Could you check a few things on this model? Use its own coordinates, in mm. A direction names the side the tool comes from. Round coordinates to 2 decimals unless told otherwise and drop trailing zeros. Write each loop counter-clockwise with the first axis right and the second up, starting at its lowest first coordinate (ties: lowest second). Pieces come first, ordered by that corner, then holes. Notation, with made-up numbers: (84.25, -31) -> (91.25, -31) arc R17 ccw to (91.25, -16) -> close; hole circle Ø3 at (84, 10). An arc over 180 degrees is marked (long way). One line per question, with ' | ' between items. Start each with the question number.
1. For pin 1 Ø4 at (x, z) = (-79.2, 57.98) entering from -Y; pin 2 Ø2.5 at (x, z) = (-120, -50) entering from +Y, each with a flat end and sliding along its axis, tell me the tip position at first contact or that it passes through.
2. Imagine slicing it at B-B, the plane y = 1. State how many separate pieces and enclosed holes the cut face has, and give its area (3 significant figures).
3. Imagine slicing it at D-D, the plane z = 4. List the corners of the cut face in (x, y) for me, and give its area (3 significant figures).
4. Thinking about a two-plate mould opening in Z: for faces 1 (the cylindrical face through (-86.498, 1.479, 64.66)), 2 (the flat face through (-63.542, 1.521, -111.609)), 3 (the flat face through (-123, 3, -26)), which applies, released by +Z, released by -Z, zero draft, split by the parting line, or undercut?
5. For faces 4 (the flat face through (-123, 0, -26)), 5 (the cylindrical face through (-67.015, 1.521, -78.745)), 6 (the flat face through (-99.133, 1.521, 63.743)), which set-ups out of +Z, -Z, +X, -X, +Y, -Y let a thin tool reach every point of the face, with its end or its side?
6. Imagine slicing it at C-C, the plane z = 28. List the corners of the cut face in (x, y) for me.
7. If I drill on line 1 along Z through (x, y) = (-78, 0.7); line 2 along X through (y, z) = (0.9, -70); line 3 along X through (y, z) = (1.95, -50), over which ranges is the centre line in solid material (lowest first)? Write a range as [from, to].
8. Imagine slicing it at A-A, the plane x = -105. List the corners of the cut face in (y, z) for me.
from build123d import *

# Parameters (mm, degrees)
SKETCH1_R               = 140
BOSS_EXTRUDE1_DEPTH     = 3
CUT_EXTRUDE1_REACH      = 5
CUT_EXTRUDE3_REACH      = 5
SKETCH19_R              = 1.5
CUT_EXTRUDE10_REACH     = 5
SKETCH25_R              = 1.5
CUT_EXTRUDE4_REACH      = 5
FILLET2_R               = 10
CUT_EXTRUDE8_DEPTH      = 1
CUT_EXTRUDE8_DEPTH_BACK = 4
CUT_EXTRUDE9_REACH      = 5
FILLET4_R               = 5
FILLET5_R               = 3


with BuildPart() as part:
    # Sketch1 → Boss-Extrude1 (new body)
    with BuildSketch(Plane(origin=(0, 0, 0), x_dir=(1, 0, 0), z_dir=(0, 1, 0))):
        Circle(SKETCH1_R)
    extrude(amount=BOSS_EXTRUDE1_DEPTH)

    # Sketch17 → Cut-Extrude1 (cut, up to next)
    with BuildSketch(Plane.XZ, mode=Mode.PRIVATE) as cut_extrude1_sk1:
        Polygon((-50, 90), (-121.24355653, 70), (-121.24355653, 140), (121.24355653, 140), (121.24355653, 70), (50, 90), align=None)
    cut_extrude1_tool1 = extrude(cut_extrude1_sk1.sketch, amount=-CUT_EXTRUDE1_REACH, mode=Mode.PRIVATE) & part.part
    add(cut_extrude1_tool1.solids().sort_by_distance((0, 0, 111.669853))[0], mode=Mode.SUBTRACT)

    # Sketch19 → Cut-Extrude3 (cut, up to next)
    with BuildSketch(Plane(origin=(0, 3, 0), x_dir=(1, 0, 0), z_dir=(0, 1, 0)), mode=Mode.PRIVATE) as cut_extrude3_sk1:
        with Locations((-79.195959493, -57.982756057)):
            Circle(SKETCH19_R)
    cut_extrude3_tool1 = extrude(cut_extrude3_sk1.sketch, amount=-CUT_EXTRUDE3_REACH, mode=Mode.PRIVATE) & part.part
    add(cut_extrude3_tool1.solids().sort_by_distance((-79.195959, 3, 57.982756))[0], mode=Mode.SUBTRACT)
    # Sketch19 → Cut-Extrude3 (cut, up to next)
    with BuildSketch(Plane(origin=(0, 3, 0), x_dir=(1, 0, 0), z_dir=(0, 1, 0)), mode=Mode.PRIVATE) as cut_extrude3_sk2:
        with Locations((-79.195959493, 57.982756057)):
            Circle(SKETCH19_R)
    cut_extrude3_tool2 = extrude(cut_extrude3_sk2.sketch, amount=-CUT_EXTRUDE3_REACH, mode=Mode.PRIVATE) & part.part
    add(cut_extrude3_tool2.solids().sort_by_distance((-79.195959, 3, -57.982756))[0], mode=Mode.SUBTRACT)
    # Sketch19 → Cut-Extrude3 (cut, up to next)
    with BuildSketch(Plane(origin=(0, 3, 0), x_dir=(1, 0, 0), z_dir=(0, 1, 0)), mode=Mode.PRIVATE) as cut_extrude3_sk3:
        with Locations((79.195959493, 57.982756057)):
            Circle(SKETCH19_R)
    cut_extrude3_tool3 = extrude(cut_extrude3_sk3.sketch, amount=-CUT_EXTRUDE3_REACH, mode=Mode.PRIVATE) & part.part
    add(cut_extrude3_tool3.solids().sort_by_distance((79.195959, 3, -57.982756))[0], mode=Mode.SUBTRACT)
    # Sketch19 → Cut-Extrude3 (cut, up to next)
    with BuildSketch(Plane(origin=(0, 3, 0), x_dir=(1, 0, 0), z_dir=(0, 1, 0)), mode=Mode.PRIVATE) as cut_extrude3_sk4:
        with Locations((79.195959493, -57.982756057)):
            Circle(SKETCH19_R)
    cut_extrude3_tool4 = extrude(cut_extrude3_sk4.sketch, amount=-CUT_EXTRUDE3_REACH, mode=Mode.PRIVATE) & part.part
    add(cut_extrude3_tool4.solids().sort_by_distance((79.195959, 3, 57.982756))[0], mode=Mode.SUBTRACT)
    # Sketch19 → Cut-Extrude3 (cut, up to next)
    with BuildSketch(Plane(origin=(0, 3, 0), x_dir=(1, 0, 0), z_dir=(0, 1, 0)), mode=Mode.PRIVATE) as cut_extrude3_sk5:
        with Locations((-57.982756057, 79.195959493)):
            Circle(SKETCH19_R)
    cut_extrude3_tool5 = extrude(cut_extrude3_sk5.sketch, amount=-CUT_EXTRUDE3_REACH, mode=Mode.PRIVATE) & part.part
    add(cut_extrude3_tool5.solids().sort_by_distance((-57.982756, 3, -79.195959))[0], mode=Mode.SUBTRACT)
    # Sketch19 → Cut-Extrude3 (cut, up to next)
    with BuildSketch(Plane(origin=(0, 3, 0), x_dir=(1, 0, 0), z_dir=(0, 1, 0)), mode=Mode.PRIVATE) as cut_extrude3_sk6:
        with Locations((57.982756057, 79.195959493)):
            Circle(SKETCH19_R)
    cut_extrude3_tool6 = extrude(cut_extrude3_sk6.sketch, amount=-CUT_EXTRUDE3_REACH, mode=Mode.PRIVATE) & part.part
    add(cut_extrude3_tool6.solids().sort_by_distance((57.982756, 3, -79.195959))[0], mode=Mode.SUBTRACT)
    # Sketch19 → Cut-Extrude3 (cut, up to next)
    with BuildSketch(Plane(origin=(0, 3, 0), x_dir=(1, 0, 0), z_dir=(0, 1, 0)), mode=Mode.PRIVATE) as cut_extrude3_sk7:
        with Locations((57.982756057, -79.195959493)):
            Circle(SKETCH19_R)
    cut_extrude3_tool7 = extrude(cut_extrude3_sk7.sketch, amount=-CUT_EXTRUDE3_REACH, mode=Mode.PRIVATE) & part.part
    add(cut_extrude3_tool7.solids().sort_by_distance((57.982756, 3, 79.195959))[0], mode=Mode.SUBTRACT)
    # Sketch19 → Cut-Extrude3 (cut, up to next)
    with BuildSketch(Plane(origin=(0, 3, 0), x_dir=(1, 0, 0), z_dir=(0, 1, 0)), mode=Mode.PRIVATE) as cut_extrude3_sk8:
        with Locations((-57.982756057, -79.195959493)):
            Circle(SKETCH19_R)
    cut_extrude3_tool8 = extrude(cut_extrude3_sk8.sketch, amount=-CUT_EXTRUDE3_REACH, mode=Mode.PRIVATE) & part.part
    add(cut_extrude3_tool8.solids().sort_by_distance((-57.982756, 3, 79.195959))[0], mode=Mode.SUBTRACT)

    # Sketch25 → Cut-Extrude10 (cut, up to next)
    with BuildSketch(Plane(origin=(0, 3, 0), x_dir=(1, 0, 0), z_dir=(0, 1, 0)), mode=Mode.PRIVATE) as cut_extrude10_sk1:
        with Locations((-120, 50)):
            Circle(SKETCH25_R)
    cut_extrude10_tool1 = extrude(cut_extrude10_sk1.sketch, amount=-CUT_EXTRUDE10_REACH, mode=Mode.PRIVATE) & part.part
    add(cut_extrude10_tool1.solids().sort_by_distance((-120, 3, -50))[0], mode=Mode.SUBTRACT)
    # Sketch25 → Cut-Extrude10 (cut, up to next)
    with BuildSketch(Plane(origin=(0, 3, 0), x_dir=(1, 0, 0), z_dir=(0, 1, 0)), mode=Mode.PRIVATE) as cut_extrude10_sk2:
        with Locations((-120, -50)):
            Circle(SKETCH25_R)
    cut_extrude10_tool2 = extrude(cut_extrude10_sk2.sketch, amount=-CUT_EXTRUDE10_REACH, mode=Mode.PRIVATE) & part.part
    add(cut_extrude10_tool2.solids().sort_by_distance((-120, 3, 50))[0], mode=Mode.SUBTRACT)

    # Sketch20 → Cut-Extrude4 (cut, up to next)
    with BuildSketch(Plane(origin=(0, 3, 0), x_dir=(1, 0, 0), z_dir=(0, 1, 0)), mode=Mode.PRIVATE) as cut_extrude4_sk1:
        Polygon((-501.142143979, 549.208792138), (-72, 120.066648158), (-50, 98.066648158), (50, 98.066648158), (72, 120.066648158), (501.142143979, 549.208792138), (501.142143979, 1763.00607254), (-501.142143979, 1763.00607254), align=None)
    cut_extrude4_tool1 = extrude(cut_extrude4_sk1.sketch, amount=-CUT_EXTRUDE4_REACH, mode=Mode.PRIVATE) & part.part
    add(cut_extrude4_tool1.solids().sort_by_distance((0, 3, -1025.283687))[0], mode=Mode.SUBTRACT)

    # Fillet2
    fillet2_edges = [part.edges().sort_by_distance(p)[0] for p in [
        (50, 1.5, -98.066648158),
        (-50, 1.5, -98.066648158),
    ]]
    fillet(fillet2_edges, radius=FILLET2_R)

    # Sketch23 → Cut-Extrude8 (cut, two sides)
    with BuildSketch(Plane(origin=(0, 3, 0), x_dir=(1, 0, 0), z_dir=(0, 1, 0))) as cut_extrude8_sk:
        with BuildLine():
            Line((257.25555619, 635.882543767), (-54.933351842, 103))
            ThreePointArc((-54.933351842, 103), (-81.898962794, 15.574433529), (-67.110613718, -74.712213204))
            Line((-67.110613718, -74.712213204), (-73.189737717, -96.367133919))
            Line((-73.189737717, -96.367133919), (-240.113193325, -690.978166206))
            Line((-240.113193325, -690.978166206), (916.492938423, -1124.527627053))
            Line((916.492938423, -1124.527627053), (1413.861687938, 202.33308292))
            Line((1413.861687938, 202.33308292), (257.25555619, 635.882543767))
        make_face()
    extrude(amount=CUT_EXTRUDE8_DEPTH, mode=Mode.SUBTRACT)
    extrude(cut_extrude8_sk.sketch, amount=-CUT_EXTRUDE8_DEPTH_BACK, mode=Mode.SUBTRACT)

    # Sketch24 → Cut-Extrude9 (cut, up to next)
    with BuildSketch(Plane(origin=(0, 3, 0), x_dir=(1, 0, 0), z_dir=(0, 1, 0)), mode=Mode.PRIVATE) as cut_extrude9_sk1:
        with BuildLine():
            Line((-87.357146899, 55.966584143), (-76.169199175, 51.304939258))
            Line((-76.169199175, 51.304939258), (-75.263305358, -50.927483501))
            Line((-75.263305358, -50.927483501), (-86.425648637, -55.578459868))
            ThreePointArc((-86.425648637, -55.578459868), (-84.491324796, -62.048707618), (-82.351900579, -68.454063088))
            Line((-82.351900579, -68.454063088), (-109.142815319, -60.933126165))
            ThreePointArc((-109.142815319, -60.933126165), (-121.247849947, 30.39669198), (-67.489752352, 105.2147011))
            ThreePointArc((-67.489752352, 105.2147011), (-78.971583679, 81.215182034), (-87.357146899, 55.966584143))
        make_face()
    cut_extrude9_tool1 = extrude(cut_extrude9_sk1.sketch, amount=-CUT_EXTRUDE9_REACH, mode=Mode.PRIVATE) & part.part
    add(cut_extrude9_tool1.solids().sort_by_distance((-97.439624, 3, -6.929648))[0], mode=Mode.SUBTRACT)

    # Fillet4
    fillet4_edges = [part.edges().sort_by_distance(p)[0] for p in [
        (-109.142815319, 1.5, 60.933126165),
        (-67.489752352, 1.5, -105.2147011),
        (-82.351900579, 1.5, 68.454063088),
    ]]
    fillet(fillet4_edges, radius=FILLET4_R)

    # Fillet5
    fillet5_edges = [part.edges().sort_by_distance(p)[0] for p in [
        (-87.357146899, 1.5, -55.966584143),
        (-76.169199175, 1.5, -51.304939258),
        (-75.263305358, 1.5, 50.927483501),
        (-86.425648637, 1.5, 55.578459868),
        (-121.24355653, 1.5, 70),
        (-72, 1.5, -120.066648158),
        (-54.933351842, 1.5, -103),
        (-69.838855295, 1.5, 84.430694855),
        (-67.110613718, 1.5, 74.712213204),
    ]]
    fillet(fillet5_edges, radius=FILLET5_R)


solid = part.part
Geometry results:
1) pin 1: stops at y = 0 | pin 2: passes through
2) separate pieces: 1 | enclosed holes: 4 | area: 4,650 mm2
3) outline: (-139.94, 0) -> (-124.94, 0) -> (-124.94, 3) -> (-139.94, 3) -> close | area: 45.0 mm2
4) face 1: undercut | face 2: released by -Z | face 3: zero draft
5) face 4: +Z, -Z, +X, -X, -Y | face 5: +X, +Y, -Y | face 6: +Y, -Y
6) outline: (-137.17, 0) -> (-121.82, 0) -> (-121.82, 3) -> (-137.17, 3) -> close
7) line 1: z = [-116.26, -91.58], [-83.58, -58.89], [-57.08, -52.4], [52.1, 57.08], [58.89, 82.14] | line 2: x = [-121.24, -103.56], [-83.13, -70.42] | line 3: x = [-130.77, -121.5], [-118.5, -114.56]
8) outline: (0, -92.6) -> (3, -92.6) -> (3, -67.82) -> (0, -67.82) -> close; (0, 62.1) -> (3, 62.1) -> (3, 74.56) -> (0, 74.56) -> close
